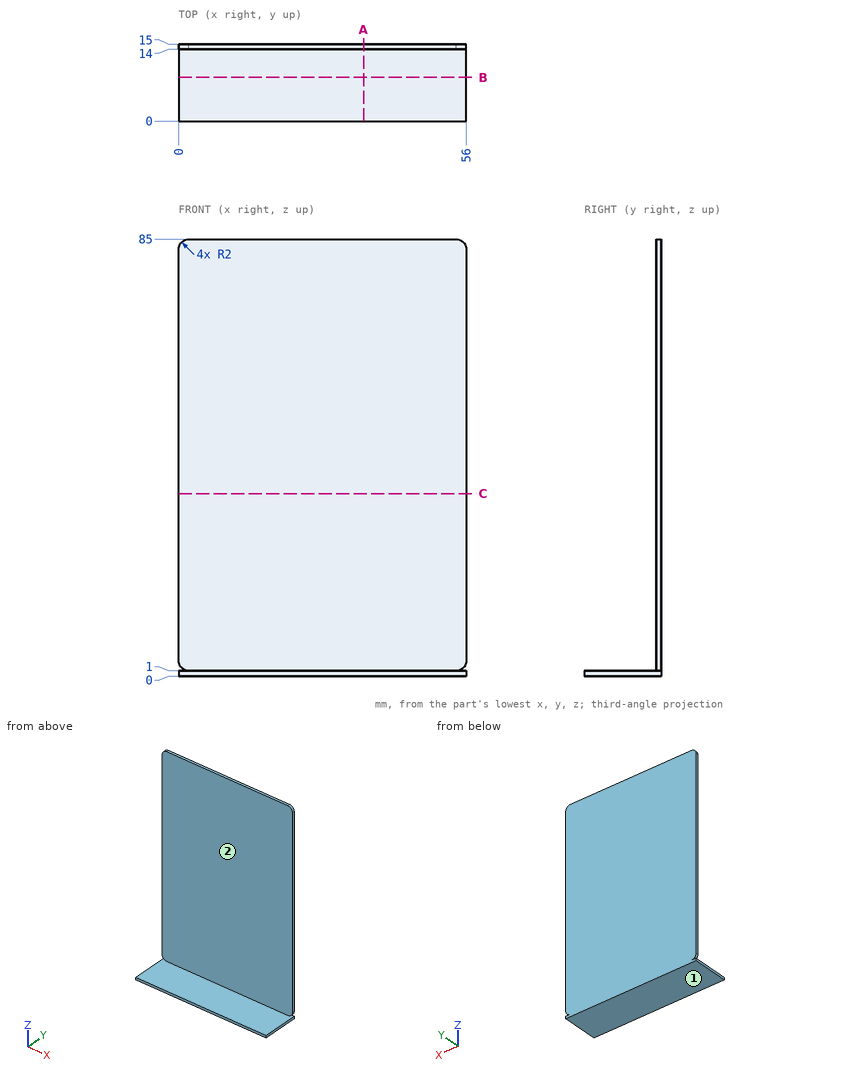
Study the drawing (mm; zero at the part's minimum x, y, z) and answer. Coordinates: 2 decimals unless noted, no trailing zeros. Loops run counter-clockwise (first coordinate to the right, second up) from the corner with the lowest first, then second, coordinate; pieces in that order, holes last. Notation, with made-up numbers: (-20.75, 88) -> (8.25, 88) arc R19 cw to (8.25, 113) -> close; hole circle Ø11 at (19.25, 44.25). An arc over 180 degrees is marked (long way). Write each question's results on one line, items separated by ' | '. Start each with the question number.
1) Find section B-B on y = 8.5. Determine the outline of the cut face in (x, z), then the cut area to 3 significant figures.
2) Consider line 1 along Y through (x, z) = (45, 75); line 2 along Z through (x, y) = (29, 2.25). Determine where each line is inside the solid, lowest interval first.
3) The mould has two halves that part along Z. Classify the marked faces 1 and 2: pulls with the +Z half, pulls with the -Z half, needs draft (parallel to the pull), parting line crosses it, or undercut.
4) Find section C-C on z = 35.5. Determine the outline of the cut face in (x, y).
5) Flat-ended cylindrical pins translate along their axes: P1, Ø1.5, axis at x = 27, z = 26.5, coming from the -Y side; P2, Ø2, axis at x = 7, y = 11.5, coming from the -Z side; P3, Ø2, axis at x = 13, y = 7, coming from the +Z side. Find the tip coordinate at first contact, or state that the pin passes through.
6) Find section A-A on x = 36. Determine the outline of the cut face in (y, z), then the cut area to 3 significant figures.
Response values:
1) outline: (0, 0) -> (56, 0) -> (56, 1) -> (0, 1) -> close | area: 56.0 mm^2
2) line 1: y = 14 to 15 | line 2: z = 0 to 1
3) face 1: pulls with the -Z half | face 2: needs draft
4) outline: (0, 14) -> (56, 14) -> (56, 15) -> (0, 15) -> close
5) P1: stops at y = 14 | P2: stops at z = 0 | P3: stops at z = 1
6) outline: (0, 0) -> (15, 0) -> (15, 85) -> (14, 85) -> (14, 1) -> (0, 1) -> close | area: 99.0 mm^2
